Verification items for this drawing (mm, ordinates from the low corner). A direction names the side the tool comes from. Coordinates: 2 decimals unless noted, no trailing zeros. Order: outer loops, then holes, each group sorted by start corner. A loop starts at its lowest first (then second) coordinate and runs counter-clockwise, first axis right, second up.
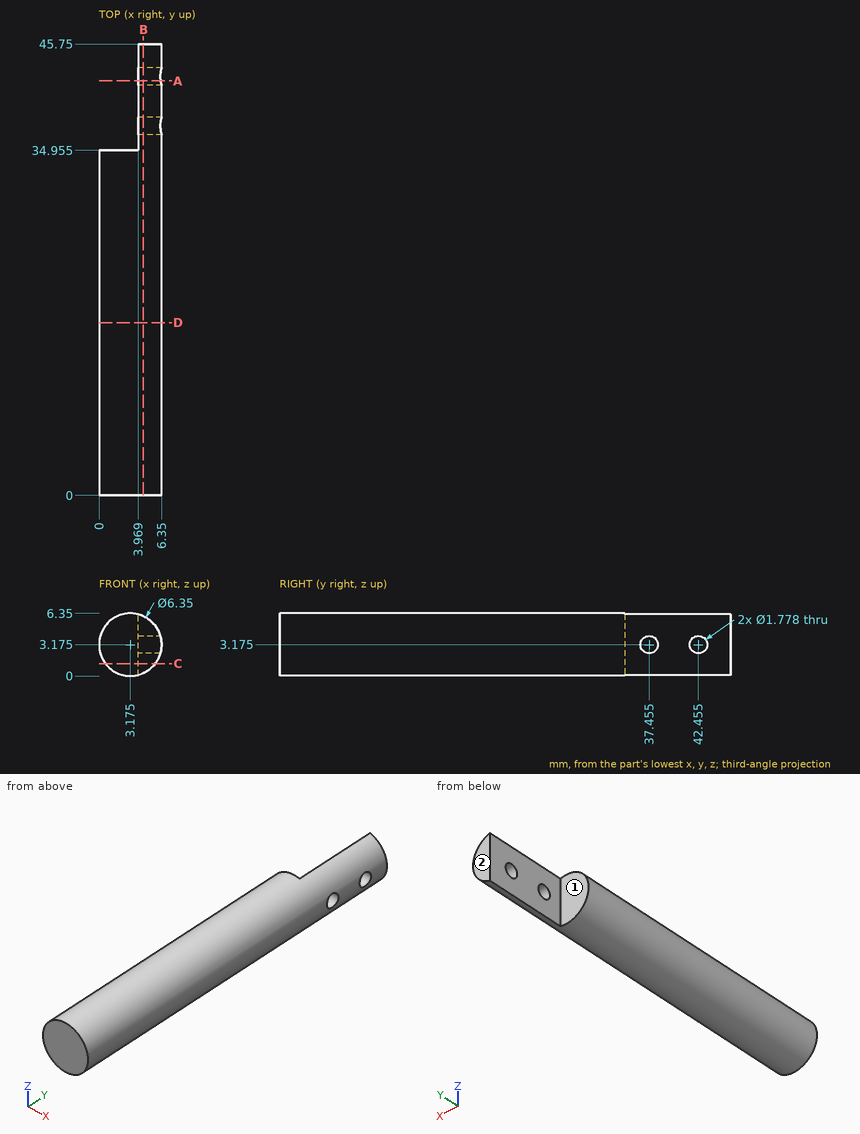
(1) Go/stop test with flat-tipped pins: P1, Ø2, axis at x = 2, y = 15.5, coming from the -Z side; P2, Ø3, axis at x = 1.5, z = 2, coming from the +Y side (3 decimals); P3, Ø3, axis at y = 42.455, z = 3.175, coming from the -X side. Record where each tip stops, or that it passes through.
Filled in:
P1: stops at z = 0
P2: stops at y = 34.955
P3: stops at x = 3.97
(2) Cross-section at C-C (z = 1.25). Enter the section's corners in (x, y) (3 decimals).
Filled in:
outline: (0.65, 0) - (5.7, 0) - (5.7, 45.75) - (3.969, 45.75) - (3.969, 34.955) - (0.65, 34.955) - close
(3) Cross-section at B-B (x = 4.5). Enter the section's corners in (y, z) (3 decimals).
Filled in:
outline: (0, 0.29) - (45.75, 0.29) - (45.75, 6.06) - (0, 6.06) - close; hole circle Ø1.778 at (37.455, 3.175); hole circle Ø1.778 at (42.455, 3.175)
(4) Cross-section at D-D (y = 17.5). Enter the section's corners in (x, z) (3 decimals).
Filled in:
outline: circle Ø6.35 at (3.175, 3.175)
(5) Tool access check on the marked faces 1 and 2. Record the directions out of +Z, -Z, +X, -X, +Y, -Y that give a thin tool (end or side, any length) a straight path to the whole face; none if there is none.
Filled in:
face 1: +Z, -Z, -X, +Y
face 2: +Z, -Z, +X, -X, +Y
(6) Cross-section at A-A (y = 42). Enter the section's corners in (x, z) (3 decimals).
Filled in:
outline: (3.969, 0.101) arc R3.175 ccw to (6.257, 2.411) - (3.969, 2.411) - close; (3.969, 3.939) - (6.257, 3.939) arc R3.175 ccw to (3.969, 6.249) - close
(7) Thickness scan on probe 1 along Y at (x, z) = (4, 3.25); probe 2 along Z at (x, y) = (4, 17.5); probe 3 along Y at (x, z) = (2, 6) (3 decimals). Record the ranges inside material, lowest first.
Filled in:
probe 1: y = 0 to 36.57, 38.34 to 41.57, 43.34 to 45.75
probe 2: z = 0.11 to 6.24
probe 3: y = 0 to 34.955
